Verification items for this drawing (mm, ordinates from the low corner). Round coordinates to 2 decimals unless told otherwise and drop trailing zeros. Order: outer loops, then holes, each group sorted by start corner. A loop starts at its lowest first (then second) coordinate and runs counter-clockwise, first axis right, second up. Notation, with made-up numbers: (19.5, 17.25) - (44.5, 17.25) arc R36 cw to (44.5, 56.25) - close; hole circle Ø8 at (71, 66). An arc over 180 degrees is marked (long way). Answer as CSV lines item,"result". Start each with the question number.
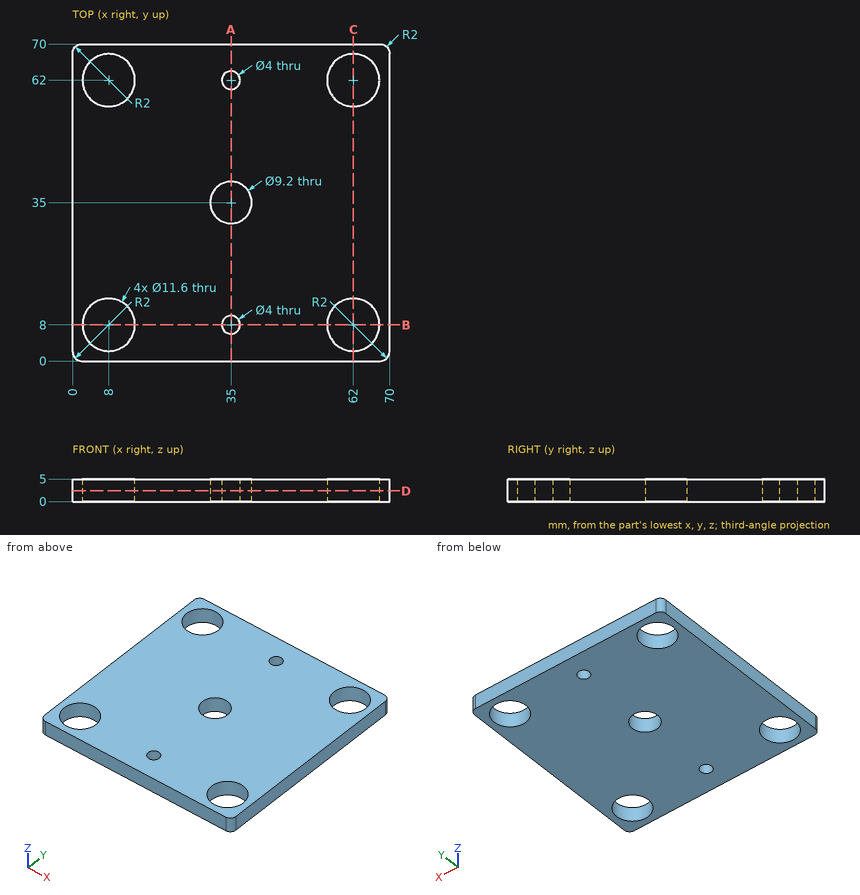
1. Section check C-C on x = 62. Record the boundary of the cut face in (y, z).
2. Section check B-B on y = 8. Record the boundary of the cut face in (x, z), plus the area to 3 significant figures.
3. Section check D-D on z = 2.4. Record the boundary of the cut face in (x, y), plus the area to 3 significant figures.
4. Section check A-A on x = 35. Record the boundary of the cut face in (y, z).
5. Go/stop test with a flat-tipped pin: pin 1 Ø5.5 at (x, y) = (35, 35) entering from +Z. Record where the tip stops, or that it passes through.
6. Thickness scan on probe 1 along Y at (x, z) = (35, 1.1); probe 2 along Y at (x, z) = (62, 3.4); probe 3 along Y at (x, z) = (5.5, 1.9). Record the ranges inside material, lowest first.
Numbers:
1,outline,"(0, 0) - (2.2, 0) - (2.2, 5) - (0, 5) - close; (13.8, 0) - (56.2, 0) - (56.2, 5) - (13.8, 5) - close; (67.8, 0) - (70, 0) - (70, 5) - (67.8, 5) - close"
2,outline,"(0, 0) - (2.2, 0) - (2.2, 5) - (0, 5) - close; (13.8, 0) - (33, 0) - (33, 5) - (13.8, 5) - close; (37, 0) - (56.2, 0) - (56.2, 5) - (37, 5) - close; (67.8, 0) - (70, 0) - (70, 5) - (67.8, 5) - close"
2,area,"214 mm2"
3,outline,"(0, 2) arc R2 ccw to (2, 0) - (68, 0) arc R2 ccw to (70, 2) - (70, 68) arc R2 ccw to (68, 70) - (2, 70) arc R2 ccw to (0, 68) - close; hole circle Ø11.6 at (8, 8); hole circle Ø11.6 at (8, 62); hole circle Ø9.2 at (35, 35); hole circle Ø4 at (35, 8); hole circle Ø4 at (35, 62); hole circle Ø11.6 at (62, 8); hole circle Ø11.6 at (62, 62)"
3,area,"4,380 mm2"
4,outline,"(0, 0) - (6, 0) - (6, 5) - (0, 5) - close; (10, 0) - (30.4, 0) - (30.4, 5) - (10, 5) - close; (39.6, 0) - (60, 0) - (60, 5) - (39.6, 5) - close; (64, 0) - (70, 0) - (70, 5) - (64, 5) - close"
5,pin 1,"passes through"
6,probe 1,"y = 0 to 6, 10 to 30.4, 39.6 to 60, 64 to 70"
6,probe 2,"y = 0 to 2.2, 13.8 to 56.2, 67.8 to 70"
6,probe 3,"y = 0 to 2.77, 13.23 to 56.77, 67.23 to 70"
